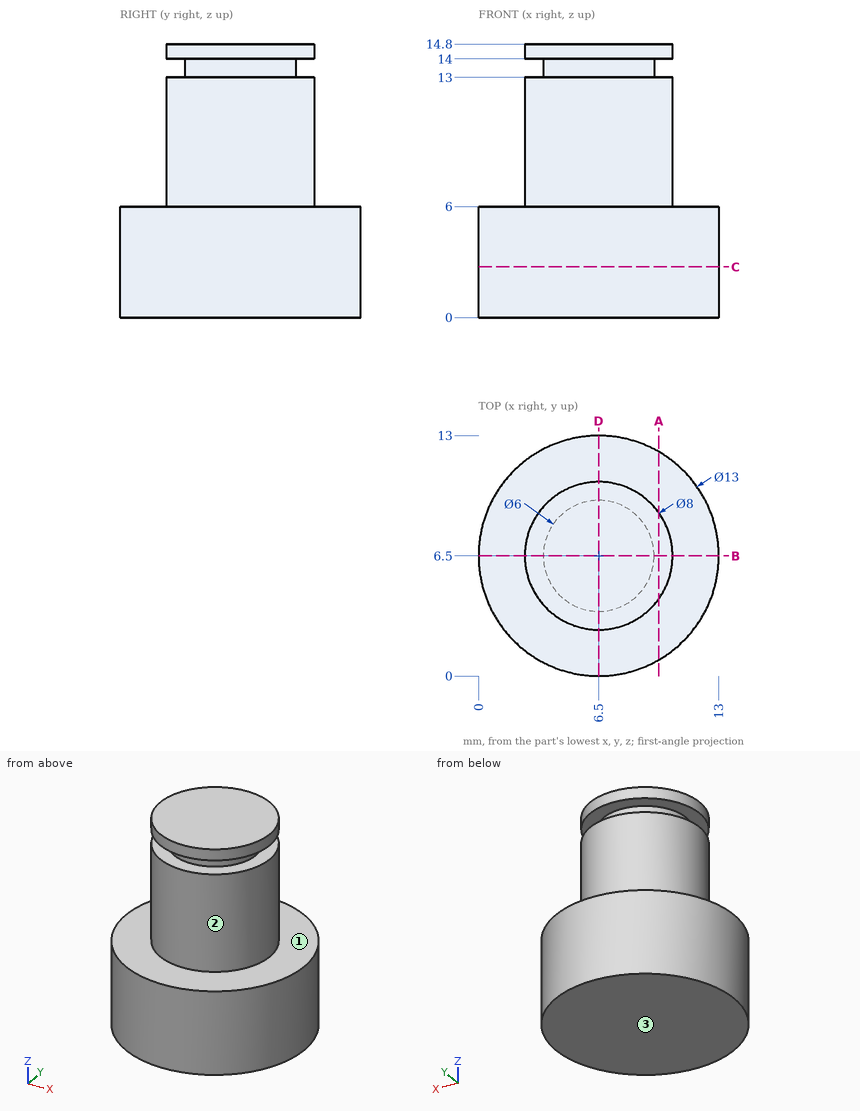
Part print with two shaded views. Sizes in mm from the minimum x, y, z corner. Round coordinates to 2 decimals unless told otherwise and drop trailing zeros. Loops run counter-clockwise (first coordinate to the right, second up) from the corner with the lowest first, then second, coordinate; pieces in that order, holes last.
1. Slice it at C-C (z = 2.75). Give the cut face in (x, y).
Solutions:
outline: circle Ø13 at (6.5, 6.5)
2. Slice it at A-A (x = 9.75). Give the cut face in (y, z).
Solutions:
outline: (0.87, 0) - (12.13, 0) - (12.13, 6) - (8.83, 6) - (8.83, 13) - (4.17, 13) - (4.17, 6) - (0.87, 6) - close; (4.17, 14) - (8.83, 14) - (8.83, 14.8) - (4.17, 14.8) - close
3. Drill centre lines: line 1 along Z through (x, y) = (3.25, 4.25); line 2 along Z through (x, y) = (1.75, 3); line 3 along Y through (x, z) = (12, 4). Where is each one in solid material? Low to high.
Solutions:
line 1: z = 0 to 13, 14 to 14.8
line 2: z = 0 to 6
line 3: y = 3.04 to 9.96
4. Flat gauge pins, fed straight in: pin 1 (4 mm diameter, centred on y = 4, z = 9, fed in from -X); pin 2 (3 mm diameter, centred on y = 10, z = 11, fed in from -X); pin 3 (1 mm diameter, centred on x = 8, z = 11.5, fed in from +Y). Where does each tip first touch, or does it go through?
Solutions:
pin 1: stops at x = 2.53
pin 2: stops at x = 3.04
pin 3: stops at y = 10.37
5. Two-plate mould, pull along Z, no slides. Class the marked faces 1, 2 and 3: pulls with the +Z half, pulls with the -Z half, needs draft (parallel to the pull), parting line crosses it, or undercut.
Solutions:
face 1: pulls with the +Z half
face 2: needs draft
face 3: pulls with the -Z half
6. Slice it at B-B (y = 6.5). Give the cut face in (x, z).
Solutions:
outline: (0, 0) - (13, 0) - (13, 6) - (10.5, 6) - (10.5, 13) - (9.5, 13) - (9.5, 14) - (10.5, 14) - (10.5, 14.8) - (2.5, 14.8) - (2.5, 14) - (3.5, 14) - (3.5, 13) - (2.5, 13) - (2.5, 6) - (0, 6) - close
